CAD build for the part. Positions are in the model's coordinates, mm. Round coordinates to 2 decimals unless told otherwise and drop trailing zeros. Write each loop counter-clockwise with the first axis right and the second up, starting at its lowest first coordinate (ties: lowest second). Pieces come first, ordered by that corner, then holes. Notation, with made-up numbers: (-23, 66.25) - (7, 66.25) arc R17 cw to (7, 81.25) - close; hole circle Ø10 at (-36.5, 53.5). An arc over 180 degrees is marked (long way). Answer in a Markdown table with one row per item.
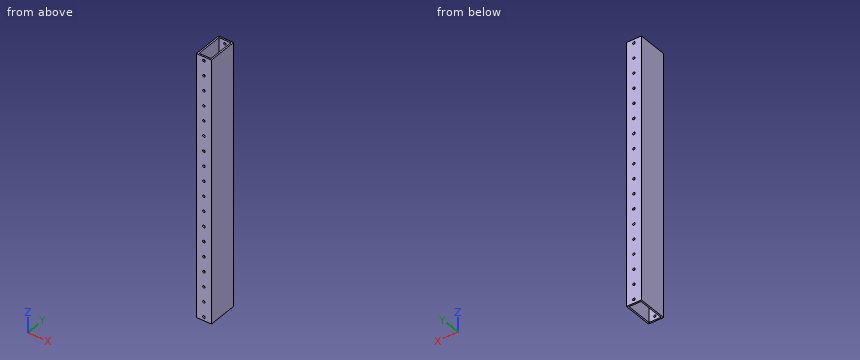
Autodesk Inventor part; units mm, degrees
ref_plane "YZ Plane" through (0, 0, 0) normal (1, 0, 0) x (0, 1, 0)
ref_plane "XZ Plane" through (0, 0, 0) normal (0, 1, 0) x (-1, 0, 0)
ref_plane "XY Plane" through (0, 0, 0) normal (0, 0, 1) x (1, 0, 0)
sketch "Sketch1" plane through (0, 0, 0) normal (0, 0, 1) x (1, 0, 0)
  line L0 (12.7, -25.4) -> (-12.7, -25.4)
  line L1 (-12.7, -25.4) -> (-12.7, 25.4)
  line L2 (-12.7, 25.4) -> (12.7, 25.4)
  line L3 (12.7, 25.4) -> (12.7, -25.4)
  line L4 (12.7, -25.4) -> (-12.7, 25.4) construction
  line L5 (-12.7, -25.4) -> (12.7, 25.4) construction
  line L6 (10.16, 22.86) -> (-10.16, 22.86)
  line L7 (-10.16, 22.86) -> (-10.16, -22.86)
  line L8 (-10.16, -22.86) -> (10.16, -22.86)
  line L9 (10.16, -22.86) -> (10.16, 22.86)
  point P0 (0, 0)
  dimension "d0" = 25.4
  dimension "d1" = 50.8
  dimension "d2" = 2.54
extrude "Extrusion1" add sketch "Sketch1" along normal mid plane 444.5
sketch "Sketch2" plane through (-12.7, 25.4, 222.25) normal (0, 1, 0) x (1, 0, 0)
  point P0 (12.7, 222.25)
  point P1 (12.7, 234.95)
  point P2 (12.7, 209.55)
  dimension "HoleOffset" = 12.7
  dimension "d6" = 12.7
hole "Hole1" at (0, 25.4, -12.7) at (0, 25.4, 12.7) direction (0, -1, 0) diameter 4.1656 end through all
pattern_linear "Rectangular Pattern1" count 31 spacing 50.8 along (0, 0, 1) of "Hole1" first direction both ways yes
properties part number "VersaFrame End Rail" material "Aluminum 6061"
Q1. Saw through at B-B on x = 6.5. List the corners of the cut face in (y, z).
Computed:
| item | result |
|---|---|
| outline | (-25.4, -222.25) - (-22.86, -222.25) - (-22.86, 222.25) - (-25.4, 222.25) - close; (22.86, -222.25) - (25.4, -222.25) - (25.4, 222.25) - (22.86, 222.25) - close |
Q2. Saw through at A-A on y = 12.5. List the corners of the cut face in (x, z).
Computed:
| item | result |
|---|---|
| outline | (-12.7, -222.25) - (-10.16, -222.25) - (-10.16, 222.25) - (-12.7, 222.25) - close; (10.16, -222.25) - (12.7, -222.25) - (12.7, 222.25) - (10.16, 222.25) - close |
Q3. Drill centre lines: line 1 (X direction, y = 24.8, z = -12.7); line 2 (X direction, y = -21, z = -134); line 3 (Y direction, x = -4.5, z = 153). Where is each one in solid material? Low to high.
Computed:
| item | result |
|---|---|
| line 1 | x = -12.7 to -2.08, 2.08 to 12.7 |
| line 2 | x = -12.7 to -10.16, 10.16 to 12.7 |
| line 3 | y = -25.4 to -22.86, 22.86 to 25.4 |
Q4. Saw through at C-C on z = 54.5. List the corners of the cut face in (x, y).
Computed:
| item | result |
|---|---|
| outline | (-12.7, -25.4) - (12.7, -25.4) - (12.7, 25.4) - (-12.7, 25.4) - close; hole (-10.16, -22.86) - (10.16, -22.86) - (10.16, 22.86) - (-10.16, 22.86) - close |
